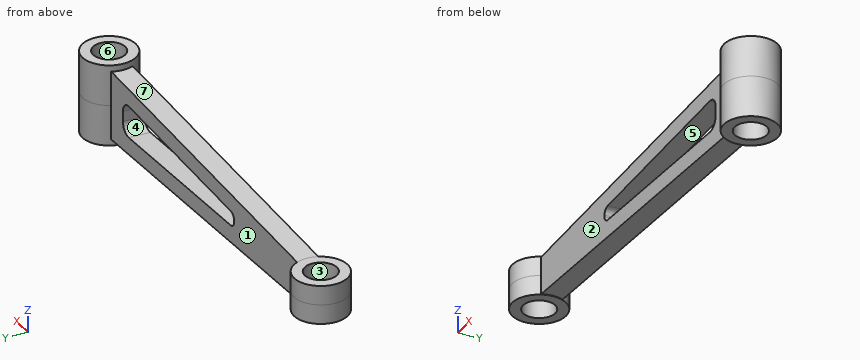
from build123d import *

# Parameters (mm, degrees)
BOSS_EXTRUDE1_DEPTH      = 10
SKETCH2_R                = 12.5
BOSS_EXTRUDE2_DEPTH      = 9
BOSS_EXTRUDE2_DEPTH_BACK = 9
SKETCH3_R                = 7.5
CUT_EXTRUDE1_DEPTH       = 26.133643284
SKETCH4_R                = 12.5
BOSS_EXTRUDE3_DEPTH      = 19
BOSS_EXTRUDE3_DEPTH_BACK = 19
SKETCH5_R                = 7.5
CUT_EXTRUDE2_DEPTH       = 39


with BuildPart() as part:
    # Sketch1 → Boss-Extrude1 (new body)
    with BuildSketch(Plane(origin=(0, 0, 0), x_dir=(1, 0, 0), z_dir=(0, 1, 0))):
        with BuildLine():
            Line((84.78, 16.133643284), (-84.78, 8.730493804))
            Line((-84.78, 8.730493804), (-84.78, 0))
            Line((-84.78, 0), (-26.81549416, 0))
            Line((-26.81549416, 0), (-26.81549416, 0.381782076))
            ThreePointArc((-26.81549416, 0.381782076), (-25.982586046, 2.456321244), (-23.946352322, 3.378926741))
            Line((-23.946352322, 3.378926741), (67.966408903, 7.391924561))
            ThreePointArc((67.966408903, 7.391924561), (71.642071119, 6.008503264), (73.18450584, 2.396683453))
            Line((73.18450584, 2.396683453), (73.18450584, 0))
            Line((73.18450584, 0), (84.78, 0))
            Line((84.78, 0), (84.78, 16.133643284))
        make_face()
    boss_extrude1 = extrude(amount=BOSS_EXTRUDE1_DEPTH)

    # Mirror1: Boss-Extrude1 across plane
    add(boss_extrude1.mirror(Plane.XY))

    # Sketch2 → Boss-Extrude2 (add, two sides)
    with BuildSketch(Plane.XY) as boss_extrude2_sk:
        with Locations((-95.28, 5)):
            Circle(SKETCH2_R)
    extrude(amount=BOSS_EXTRUDE2_DEPTH)
    extrude(boss_extrude2_sk.sketch, amount=-BOSS_EXTRUDE2_DEPTH_BACK)

    # Sketch3 → Cut-Extrude1 (cut, through all)
    with BuildSketch(Plane.XY.offset(9)):
        with Locations((-95.28, 5)):
            Circle(SKETCH3_R)
    extrude(amount=-CUT_EXTRUDE1_DEPTH, mode=Mode.SUBTRACT)

    # Sketch4 → Boss-Extrude3 (add, two sides)
    with BuildSketch(Plane.XY) as boss_extrude3_sk:
        with Locations((95.28, 5)):
            Circle(SKETCH4_R)
    extrude(amount=BOSS_EXTRUDE3_DEPTH)
    extrude(boss_extrude3_sk.sketch, amount=-BOSS_EXTRUDE3_DEPTH_BACK)

    # Sketch5 → Cut-Extrude2 (cut, through all)
    with BuildSketch(Plane.XY.offset(19)):
        with Locations((95.28, 5)):
            Circle(SKETCH5_R)
    extrude(amount=-CUT_EXTRUDE2_DEPTH, mode=Mode.SUBTRACT)


solid = part.part
The listing builds one solid part. Answer for the finished solid, in the listing's coordinates (mm). Face numbers are marked on the shaded views. A direction names the side the tool comes from. Round coordinates to 2 decimals unless told otherwise and drop trailing zeros. Order: outer loops, then holes, each group sorted by start corner. A loop starts at its lowest first (then second) coordinate and runs counter-clockwise, first axis right, second up. Notation, with made-up numbers: (62.25, 62.25) -> (79.25, 62.25) arc R18 cw to (79.25, 90.25) -> close; hole circle Ø6 at (63, 31). An arc over 180 degrees is marked (long way). Write each question's results on one line, items separated by ' | '. Start each with the question number.
Q1. Which of the six approach directions +Z, -Z, +X, -X, +Y, -Y give full straight-line access (tool end or side, diameter ignored) to the marked faces 1, 2, 3 and 4?
Q2. Each of these flat-tipped pins is pushed along its axis until it touches: pin 1 (1 mm diameter, centred on x = -13, y = 12, fed in from -Z); pin 2 (4 mm diameter, centred on x = -1, y = 6, fed in from -Z); pin 3 (1 mm diameter, centred on y = -4.5, z = 0, fed in from -X); pin 4 (16 mm diameter, centred on x = 7, z = -6.5, fed in from +Y). Where does it stop, or does it pass through?
Q3. Find section D-D (z = 13.5). Determine the outline of the cut face in (x, y).
Q4. Find section B-B (y = 5). Determine the outline of the cut face in (x, z), then the cut area to 3 significant figures.
Q5. Find section A-A (x = -95.28). Determine the outline of the cut face in (y, z), then the cut area to 3 significant figures.
Q6. The mould has two halves that part along Z. Classify the marked faces 5, 6 and 7: pulls with the +Z half, pulls with the -Z half, needs draft (parallel to the pull), parting line crosses it, or undercut.
Q7. Find section C-C (y = -4.75). Determine the outline of the cut face in (x, z), then the cut area to 3 significant figures.
Q8. Straight lines are drawn through the part: probe 1 along Y at (x, z) = (95, 5); probe 2 along Z at (x, y) = (28, 7); probe 3 along Y at (x, z) = (-98, 1). For each, find the intervals that lie inside material, in ascending order. Write a range as from..to.
Worked answers:
1) face 1: +Z, -Z, +Y | face 2: +Z, -Z, -Y | face 3: +Z, -Z | face 4: +Y, -Y
2) pin 1: passes through | pin 2: stops at z = -12.48 | pin 3: stops at x = -103.95 | pin 4: stops at y = 10
3) outline: (24.46, 0) -> (83.82, 0) arc R12.5 ccw (long way) to (83.82, 10) -> (24.46, 10) -> close; hole circle Ø15 at (95.28, 5)
4) outline: (-107.78, -9) -> (-102.78, -9) -> (-102.78, 9) -> (-107.78, 9) -> close; (-87.78, -9) -> (-82.78, -9) -> (-82.78, -8.82) -> (82.78, -16.05) -> (82.78, -19) -> (87.78, -19) -> (87.78, 19) -> (82.78, 19) -> (82.78, 16.05) -> (-82.78, 8.82) -> (-82.78, 9) -> (-87.78, 9) -> close; (102.78, -19) -> (107.78, -19) -> (107.78, 19) -> (102.78, 19) -> close; hole (-26.82, -0.38) arc R3 ccw to (-23.95, -3.38) -> (67.97, -7.39) arc R5 ccw to (73.18, -2.4) -> (73.18, 2.4) arc R5 ccw to (67.97, 7.39) -> (-23.95, 3.38) arc R3 ccw to (-26.82, 0.38) -> close | area: 3,600 mm2
5) outline: (-7.5, -9) -> (-2.5, -9) -> (-2.5, 9) -> (-7.5, 9) -> close; (12.5, -9) -> (17.5, -9) -> (17.5, 9) -> (12.5, 9) -> close | area: 180 mm2
6) face 5: undercut | face 6: needs draft | face 7: pulls with the +Z half
7) outline: (-103.1, -9) -> (-87.46, -9) -> (-87.46, 9) -> (-103.1, 9) -> close; (87.46, -19) -> (103.1, -19) -> (103.1, 19) -> (87.46, 19) -> close | area: 876 mm2
8) probe 1: y = -7.5..-2.49, 12.49..17.5 | probe 2: z = -13.65..-5.65, 5.65..13.65 | probe 3: y = -7.2..-1.99, 11.99..17.2
